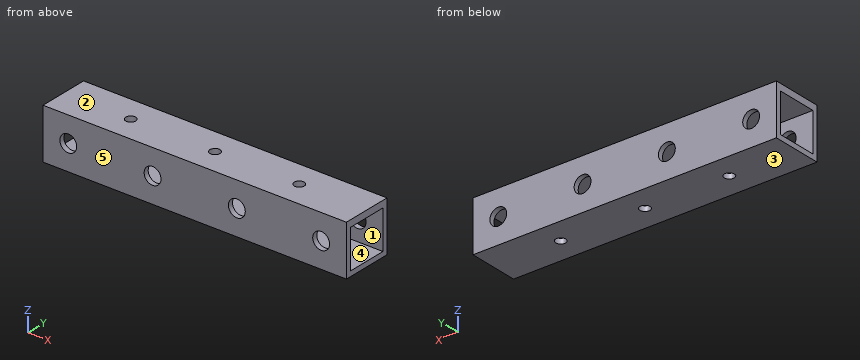
from build123d import *

# Parameters (mm, degrees)
MEMBER_15_15_1_5_1_DEPTH = 90
SKETCH_3_R               = 2.5
CUT_EXTRUDE_1_DEPTH      = 92.549167118
SKETCH_4_R               = 1.5
CUT_EXTRUDE_2_DEPTH      = 92.549167118


with BuildPart() as part:
    # Sketch1 → Member 15 _15_ 1.5_1 (new body)
    with BuildSketch(Plane(origin=(0, 0, 0), x_dir=(0, 0, -1), z_dir=(1, 0, 0))):
        Polygon((-6, -7.5), (6, -7.5), (7.5, -7.5), (7.5, -6), (7.5, 6), (7.5, 7.5), (6, 7.5), (-6, 7.5), (-7.5, 7.5), (-7.5, 6), (-7.5, -6), (-7.5, -7.5), align=None)
        Polygon((-4, -6), (4, -6), (6, -6), (6, -3.5), (6, 3.5), (6, 6), (3.5, 6), (-3.5, 6), (-5.5, 6), (-5.5, 3.5), (-5.5, -3.5), (-5.5, -6), align=None, mode=Mode.SUBTRACT)
    extrude(amount=MEMBER_15_15_1_5_1_DEPTH)

    # 草图3 → 切除-拉伸1 (cut, through all)
    with BuildSketch(Plane(origin=(0, 7.5, 0), x_dir=(1, 0, 0), z_dir=(0, 1, 0))):
        with Locations(Location((7.5, 0, 0), (0, 0, 270))):
            Circle(SKETCH_3_R)
        with Locations(Location((32.5, 0, 0), (0, 0, 270))):
            Circle(SKETCH_3_R)
        with Locations(Location((57.5, 0, 0), (0, 0, 270))):
            Circle(SKETCH_3_R)
        with Locations(Location((82.5, 0, 0), (0, 0, 270))):
            Circle(SKETCH_3_R)
    extrude(amount=-CUT_EXTRUDE_1_DEPTH, mode=Mode.SUBTRACT)

    # 草图4 → 切除-拉伸2 (cut, through all)
    with BuildSketch(Plane.XY.offset(7.5)):
        with Locations((45, 0)):
            Circle(SKETCH_4_R)
        with Locations((20, 0)):
            Circle(SKETCH_4_R)
        with Locations((70, 0)):
            Circle(SKETCH_4_R)
    extrude(amount=-CUT_EXTRUDE_2_DEPTH, mode=Mode.SUBTRACT)


solid = part.part
CAD build for the part. Positions are in the model's coordinates, mm. Face numbers are marked on the shaded views. A direction names the side the tool comes from. Coordinates: 2 decimals unless noted, no trailing zeros. Loops run counter-clockwise (first coordinate to the right, second up) from the corner with the lowest first, then second, coordinate; pieces in that order, holes last. Notation, with made-up numbers: (-25, 79) -> (0, 79) arc R13 ccw to (0, 87) -> close; hole circle Ø6 at (-13.5, 76.5). An arc over 180 degrees is marked (long way). One line per item, written item: value.
1. Which spindle directions (+Z, -Z, +X, -X, +Y, -Y) get a long thin tool onto all of the face, cutting with end or side? Do the marked faces 1 and 2. Say none if no direction does.
Answers:
face 1: +X, -X
face 2: +Z, +X, -X, +Y, -Y
2. Slice it at B-B on z = -3.25. Write the cut outline in (x, y), and give its area (3 significant figures).
Answers:
outline: (0, -7.5) -> (90, -7.5) -> (90, -6) -> (0, -6) -> close; (0, 6) -> (90, 6) -> (90, 7.5) -> (0, 7.5) -> close
area: 270 mm^2
3. Slice it at C-C on x = 13. Write the cut outline in (y, z), and give its area (3 significant figures).
Answers:
outline: (-7.5, -7.5) -> (7.5, -7.5) -> (7.5, 7.5) -> (-7.5, 7.5) -> close; hole (-6, -6) -> (6, -6) -> (6, 5.5) -> (-6, 5.5) -> close
area: 87.0 mm^2
4. Drill centre lines: line 1 (X direction, y = -6.9, z = 0); line 2 (Y direction, x = 29, z = 3.75); line 3 (Z direction, x = 81.5, y = -5.75). Where is each one in solid material? Low to high. Write a range as [from, to].
Answers:
line 1: x = [0, 5], [10, 30], [35, 55], [60, 80], [85, 90]
line 2: y = [-7.5, -6], [6, 7.5]
line 3: z = [-7.5, -6], [5.5, 7.5]
5. Pull direction Z, two halves, no side cores. Call the marked faces 3, 4 and 5: pulls with the +Z half, pulls with the -Z half, needs draft (parallel to the pull), parting line crosses it, or undercut.
Answers:
face 3: pulls with the -Z half
face 4: undercut
face 5: needs draft
6. Slice it at A-A on y = 4.5. Write the cut outline in (x, z), and give its area (3 significant figures).
Answers:
outline: (0, -7.5) -> (90, -7.5) -> (90, -6) -> (0, -6) -> close; (0, 5.5) -> (90, 5.5) -> (90, 7.5) -> (0, 7.5) -> close
area: 315 mm^2
7. Slice it at D-D on y = 0. Give the number of separate pieces and of enclosed holes in the cut face, and give its area (4 significant figures).
Answers:
separate pieces: 8
enclosed holes: 0
area: 283.5 mm^2
